For this review, use the dimensioned drawing (mm, ordinates from the lowest corner) and the shaded views. Coordinates: 2 decimals unless noted, no trailing zeros. Loops run counter-clockwise (first coordinate to the right, second up) from the corner with the lowest first, then second, coordinate; pieces in that order, holes last. Notation, with made-up numbers: M 83.5,-22 L 123.5,-22 A19 cw 123.5,-6 Z; hole C 50.5,86.25 d9. An arc over 180 degrees is marked long. Use CSV: the item, a comma, the result in double quotes. Start each with the question number.
1. Add section A-A, the plane x = 19.05. Write out the cut boundary in (y, z) (1 decimal).
2. Add section B-B, the plane z = 1.2. State how many separate pieces and enclosed holes the cut face has, then the cut area to 3 significant figures.
3. Add section C-C, the plane x = 34. Write out the cut boundary in (y, z) (1 decimal), then the cut area to 3 significant figures.
4. For L1, parallel to Y at x = 31.75, z = 1; L2, parallel to Y at x = 33, z = 2.9, list the stretches that pass through material, from the lowest coordinate up.
5. Clearance check with flat-ended pins moving along their axes: P1, Ø6, axis at x = 31.75, y = 41.275, coming from the -Z side; P2, Ø8, axis at x = 31.75, y = 9.525, coming from the +Z side (1 decimal). State where each tip first meets the part, or that it passes through.
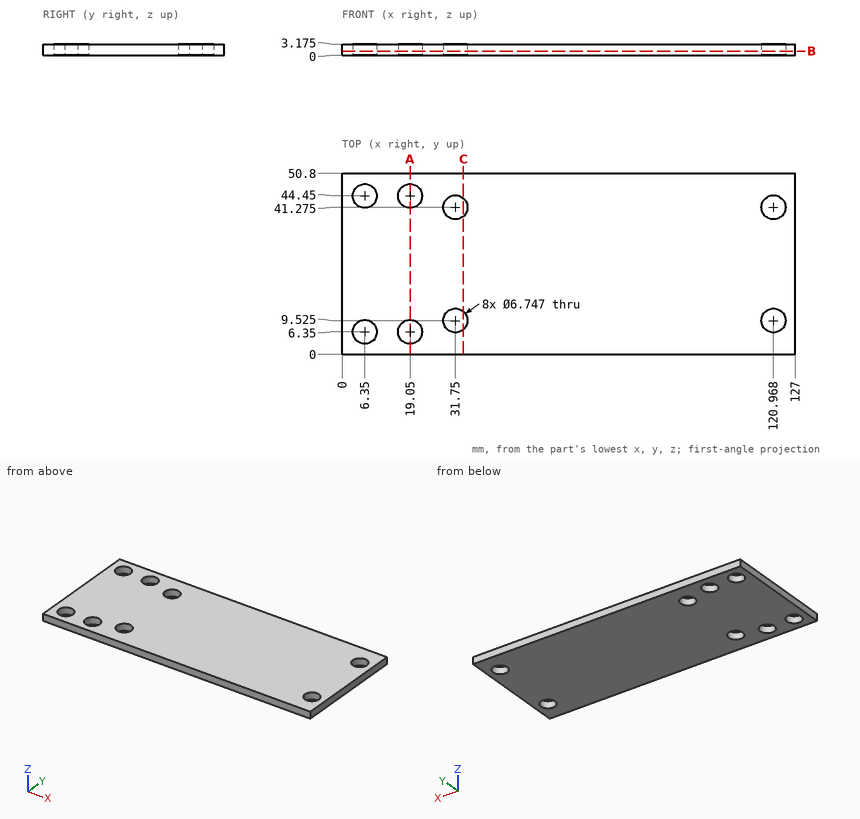
Computed:
1,outline,"M 0,0 L 3,0 L 3,3.2 L 0,3.2 Z; M 9.7,0 L 41.1,0 L 41.1,3.2 L 9.7,3.2 Z; M 47.8,0 L 50.8,0 L 50.8,3.2 L 47.8,3.2 Z"
2,separate pieces,"1"
2,enclosed holes,"8"
2,area,"6,170 mm^2"
3,outline,"M 0,0 L 7,0 L 7,3.2 L 0,3.2 Z; M 12,0 L 38.8,0 L 38.8,3.2 L 12,3.2 Z; M 43.8,0 L 50.8,0 L 50.8,3.2 L 43.8,3.2 Z"
3,area,"129 mm^2"
4,L1,"y = 0 to 6.15, 12.9 to 37.9, 44.65 to 50.8"
4,L2,"y = 0 to 6.39, 12.66 to 38.14, 44.41 to 50.8"
5,P1,"passes through"
5,P2,"stops at z = 3.2"
